Design review of the part built by this model. Coordinates are the model's own, in mm. A direction names the side the tool comes from. Give positions to 0.01 mm unless a question says otherwise; leave off trailing zeros. Write each loop counter-clockwise with the first axis right and the second up, starting at its lowest first coordinate (ties: lowest second). Pieces come first, ordered by that corner, then holes. Notation, with made-up numbers: (-14.5, 57.25) -> (12.5, 57.25) arc R25 cw to (12.5, 85.25) -> close; hole circle Ø7 at (1, 82.5). An arc over 180 degrees is marked (long way). Put each result on its own line as item: value. Start each with the question number.
from build123d import *

# Parameters (mm, degrees)
CROQUIS1_R              = 1
CROQUIS1_W              = 23.597249427
CROQUIS1_H              = 15.06
CROQUIS1_R_2            = 4.2
SALIENTE_EXTRUIR1_DEPTH = 3


with BuildPart() as part:
    # Croquis1 → Saliente-Extruir1 (new body)
    with BuildSketch(Plane.XY):
        Polygon((-333.002689238, 38.183153475), (-318.486974952, 38.183153475), (-318.486974952, 47.861153475), (-315.486974952, 47.861153475), (-315.486974952, 57.539153475), (-318.486974952, 57.539153475), (-318.486974952, 67.217153475), (-315.486974952, 67.217153475), (-315.486974952, 78.217153475), (-318.486974952, 78.217153475), (-323.486974952, 78.217153475), (-323.486974952, 81.417153475), (-328.486974952, 81.417153475), (-328.486974952, 78.217153475), (-410.096974952, 78.217153475), (-410.096974952, 81.417153475), (-415.096974952, 81.417153475), (-415.096974952, 78.217153475), (-420.096974952, 78.217153475), (-423.096974952, 78.217153475), (-423.096974952, 67.217153475), (-420.096974952, 67.217153475), (-420.096974952, 57.539153475), (-423.096974952, 57.539153475), (-423.096974952, 47.861153475), (-420.096974952, 47.861153475), (-420.096974952, 38.183153475), (-405.581260666, 38.183153475), (-405.581260666, 41.183153475), (-391.06554638, 41.183153475), (-391.06554638, 38.183153475), (-376.549832095, 38.183153475), (-376.549832095, 41.183153475), (-362.034117809, 41.183153475), (-362.034117809, 38.183153475), (-347.518403523, 38.183153475), (-347.518403523, 41.183153475), (-333.002689238, 41.183153475), align=None)
        with Locations((-399.183395748, 46.300153475)):
            Circle(CROQUIS1_R, mode=Mode.SUBTRACT)
        with Locations((-387.833395749, 58.200153475)):
            Rectangle(CROQUIS1_W, CROQUIS1_H, mode=Mode.SUBTRACT)
        with Locations((-376.483395748, 46.300153475)):
            Circle(CROQUIS1_R, mode=Mode.SUBTRACT)
        with Locations((-344.743963788, 58.200153475)):
            Circle(CROQUIS1_R_2, mode=Mode.SUBTRACT)
        with Locations((-399.183395748, 70.100153475)):
            Circle(CROQUIS1_R, mode=Mode.SUBTRACT)
        with Locations((-376.483395748, 70.100153475)):
            Circle(CROQUIS1_R, mode=Mode.SUBTRACT)
    extrude(amount=SALIENTE_EXTRUIR1_DEPTH)


solid = part.part
Q1. To check wall thickness, follow probe 1 along X at (y, z) = (58, 2.7); probe 2 along Y at (x, z) = (-391, 1.3); probe 3 along Y at (x, z) = (-392, 0.35). State the ranges of each line that lie inside material, in increasing order. Write a range as from..to.
Q2. For pin 1 (0.9 mm diameter, centred on x = -371, z = 1, fed in from -Y); pin 2 (1.5 mm diameter, centred on x = -317, z = 1.5, fed in from -Y); pin 3 (0.9 mm diameter, centred on x = -385, z = 1, fed in from +Y), all flat-tipped, find the tip position at first contact; note any pin that passes through.
Q3. Machinability: for faces 5 (the face through (-388, 65.73, 1)), 6 (the face through (-328.487, 80, 1)), 7 (the face through (-422, 67.217, 1)), 8 (the face through (-405.581, 40, 1)), which of the approach directions +Z, -Z, +X, -X, +Y, -Y give a long, thin tool a straight path to every point of the face, cutting with its end or side? Answer none if there is none.
Q4. Take a section at D-D on z = 1.85. State how many separate pieces and enclosed holes the cut face has, then the cut area to 3 significant figures.
Q5. Take a section at B-B on y = 59.5. Give the boundary of the cut face in (x, z).
Q6. Take a section at A-A on y = 53. Give the boundary of the cut face in (x, z), then the cut area to 3 significant figures.
Q7. Take a section at C-C on x = -368. Give the boundary of the cut face in (y, z).
Q8. Mouldability with a two-part tool opening along X and no side actions: class faces 1 (the face through (-370, 60, 0)), 2 (the face through (-400.182, 70.144, 1.479)), 3 (the face through (-333.003, 40, 1)), 4 (the face through (-415.097, 80, 1)) as +X half, -X half, draft (parallel to the pull), parting line (faces both ways), or undercut.
Result:
1. probe 1: x = -420.1..-399.63, -376.03..-348.94, -340.55..-318.49
1. probe 2: y = 38.18..50.67, 65.73..78.22
1. probe 3: y = 41.18..50.67, 65.73..78.22
2. pin 1: stops at y = 41.18
2. pin 2: stops at y = 47.86
2. pin 3: stops at y = 78.22
3. face 5: +Z, -Z
3. face 6: +Z, -Z, +Y
3. face 7: +Z, -Z, -X
3. face 8: +Z, -Z, -Y
4. separate pieces: 1
4. enclosed holes: 6
4. area: 3,670 mm^2
5. outline: (-420.1, 0) -> (-399.63, 0) -> (-399.63, 3) -> (-420.1, 3) -> close; (-376.03, 0) -> (-348.74, 0) -> (-348.74, 3) -> (-376.03, 3) -> close; (-340.75, 0) -> (-318.49, 0) -> (-318.49, 3) -> (-340.75, 3) -> close
6. outline: (-423.1, 0) -> (-399.63, 0) -> (-399.63, 3) -> (-423.1, 3) -> close; (-376.03, 0) -> (-315.49, 0) -> (-315.49, 3) -> (-376.03, 3) -> close
6. area: 252 mm^2
7. outline: (41.18, 0) -> (78.22, 0) -> (78.22, 3) -> (41.18, 3) -> close
8. face 1: draft
8. face 2: undercut
8. face 3: undercut
8. face 4: -X half
